from build123d import *

# Parameters (mm, degrees)
SKETCH_1_R          = 30
EXTRUDE_1_DEPTH     = 10
SKETCH_2_R          = 40
EXTRUDE_2_DEPTH     = 60
CUT_EXTRUDE_START   = -40
SKETCH_3_R          = 75
CUT_EXTRUDE_1_DEPTH = 40
CUT_EXTRUDE_2_DEPTH = 10


with BuildPart() as part:
    # Sketch 1 → Extrude 1 (new body)
    with BuildSketch(Plane(origin=(0, 0, 0), x_dir=(1, 0, 0), z_dir=(0, 1, 0))):
        with BuildLine():
            Line((-500, -450), (500, -450))
            ThreePointArc((500, -450), (570.710678119, -420.710678119), (600, -350))
            Line((600, -350), (600, 350))
            ThreePointArc((600, 350), (570.710678119, 420.710678119), (500, 450))
            Line((500, 450), (-500, 450))
            ThreePointArc((-500, 450), (-570.710678119, 420.710678119), (-600, 350))
            Line((-600, 350), (-600, -350))
            ThreePointArc((-600, -350), (-570.710678119, -420.710678119), (-500, -450))
        make_face()
        with Locations(Location((-500, 350, 0), (0, 0, 270))):
            Circle(SKETCH_1_R, mode=Mode.SUBTRACT)
        with Locations(Location((500, 350, 0), (0, 0, 270))):
            Circle(SKETCH_1_R, mode=Mode.SUBTRACT)
        with Locations(Location((-500, -350, 0), (0, 0, 270))):
            Circle(SKETCH_1_R, mode=Mode.SUBTRACT)
        with Locations(Location((500, -350, 0), (0, 0, 270))):
            Circle(SKETCH_1_R, mode=Mode.SUBTRACT)
    extrude(amount=EXTRUDE_1_DEPTH)

    # Sketch 2 → Extrude 2 (add)
    with BuildSketch(Plane(origin=(0, 10, 0), x_dir=(1, 0, 0), z_dir=(0, 1, 0))):
        with BuildLine():
            Line((600, -350), (600, 350))
            ThreePointArc((600, 350), (570.710678119, 420.710678119), (500, 450))
            Line((500, 450), (-500, 450))
            ThreePointArc((-500, 450), (-570.710678119, 420.710678119), (-600, 350))
            Line((-600, 350), (-600, -350))
            ThreePointArc((-600, -350), (-570.710678119, -420.710678119), (-500, -450))
            Line((-500, -450), (500, -450))
            ThreePointArc((500, -450), (570.710678119, -420.710678119), (600, -350))
        make_face()
        with Locations(Location((-500, 350, 0), (0, 0, 270))):
            Circle(SKETCH_2_R, mode=Mode.SUBTRACT)
        with Locations(Location((-500, -350, 0), (0, 0, 270))):
            Circle(SKETCH_2_R, mode=Mode.SUBTRACT)
        with Locations(Location((500, -350, 0), (0, 0, 270))):
            Circle(SKETCH_2_R, mode=Mode.SUBTRACT)
        with Locations(Location((500, 350, 0), (0, 0, 270))):
            Circle(SKETCH_2_R, mode=Mode.SUBTRACT)
    extrude(amount=EXTRUDE_2_DEPTH)

    # Sketch 3 → Cut-Extrude 1 (cut)
    with BuildSketch(Plane(origin=(0, 70, 0), x_dir=(1, 0, 0), z_dir=(0, 1, 0)).offset(CUT_EXTRUDE_START)):
        with BuildLine():
            Line((600, -350), (600, 350))
            ThreePointArc((600, 350), (570.710678119, 420.710678119), (500, 450))
            Line((500, 450), (-500, 450))
            ThreePointArc((-500, 450), (-570.710678119, 420.710678119), (-600, 350))
            Line((-600, 350), (-600, -350))
            ThreePointArc((-600, -350), (-570.710678119, -420.710678119), (-500, -450))
            Line((-500, -450), (500, -450))
            ThreePointArc((500, -450), (570.710678119, -420.710678119), (600, -350))
        make_face()
        with Locations(Location((-500, 350, 0), (0, 0, 270))):
            Circle(SKETCH_3_R, mode=Mode.SUBTRACT)
        with Locations(Location((-500, -350, 0), (0, 0, 270))):
            Circle(SKETCH_3_R, mode=Mode.SUBTRACT)
        with Locations(Location((500, 350, 0), (0, 0, 270))):
            Circle(SKETCH_3_R, mode=Mode.SUBTRACT)
        with Locations(Location((500, -350, 0), (0, 0, 270))):
            Circle(SKETCH_3_R, mode=Mode.SUBTRACT)
    extrude(amount=CUT_EXTRUDE_1_DEPTH, mode=Mode.SUBTRACT)

    # Sketch 7 → Cut-Extrude 2 (cut)
    with BuildSketch(Plane(origin=(0, 70, 0), x_dir=(1, 0, 0), z_dir=(0, 1, 0))):
        with BuildLine():
            Line((-425, 346.5), (-445, 346.5))
            ThreePointArc((-445, 346.5), (-448.5, 350), (-445, 353.5))
            Line((-445, 353.5), (-425, 353.5))
            ThreePointArc((-425, 353.5), (-421.5, 350), (-425, 346.5))
        make_face()
        with BuildLine():
            Line((575, 346.5), (555, 346.5))
            ThreePointArc((555, 346.5), (551.5, 350), (555, 353.5))
            Line((555, 353.5), (575, 353.5))
            ThreePointArc((575, 353.5), (578.5, 350), (575, 346.5))
        make_face()
        with BuildLine():
            Line((575, -353.5), (555, -353.5))
            ThreePointArc((555, -353.5), (551.5, -350), (555, -346.5))
            Line((555, -346.5), (575, -346.5))
            ThreePointArc((575, -346.5), (578.5, -350), (575, -353.5))
        make_face()
        with BuildLine():
            Line((-425, -353.5), (-445, -353.5))
            ThreePointArc((-445, -353.5), (-448.5, -350), (-445, -346.5))
            Line((-445, -346.5), (-425, -346.5))
            ThreePointArc((-425, -346.5), (-421.5, -350), (-425, -353.5))
        make_face()
    extrude(amount=-CUT_EXTRUDE_2_DEPTH, mode=Mode.SUBTRACT)


solid = part.part
Can you work these out from the model? Positions are in its coordinate system, mm. A direction names the side the tool comes from. Coordinates: 2 decimals unless noted, no trailing zeros. Write each loop counter-clockwise with the first axis right and the second up, starting at its lowest first coordinate (ties: lowest second). Pieces come first, ordered by that corner, then holes. Notation, with made-up numbers: (33, 65.5) - (73, 65.5) arc R11 cw to (73, 70.5) - close; hole circle Ø7 at (-33, 1). An arc over 180 degrees is marked (long way). Return JSON: item names as keys, results as strings. Group by question number.
Item 1: If we section it at D-D (z = 29): Write out the boundary of the cut face in (x, y).
Item 2: Which directions (+Z, -Z, +X, -X, +Y, -Y) give clear straight access to the entire face, cutting with the end or side of a thin tool? Please do faces 5 (the face through (-600, 15, -5)), 6 (the face through (563.24, 49.72, -309.68)).
Item 3: We'd pull the mould along X, two halves only. Please class faces 1 (the face through (-571.484, 14.79, 419.929)), 2 (the face through (-529.287, 4.93, 343.497)), 3 (the face through (571.484, 14.79, -419.929)), 4 (the face through (-7, 15, 450)): pulls with the +X half, pulls with the -X half, needs draft (parallel to the pull), parting line crosses it, or undercut.
Item 4: If we section it at B-B (z = 366): Write out the boundary of the cut face in (x, y), then the cut area to 3 significant figures.
Item 5: If we section it at A-A (y = 48): Write out the boundary of the cut face in (x, z).
Item 6: Please list where these lines run through material, in increasing order: probe 1 along X at (y, z) = (5.25, -350); probe 2 along X at (y, z) = (53, 350); probe 3 along X at (y, z) = (23, -350).
Item 7: I'm going to push flat-ended pins straight in: pin 1 Ø11 at (x, y) = (-432.5, 63) entering from -Z; pin 2 Ø8 at (x, z) = (299.5, -59.5) entering from +Y; pin 3 Ø10 at (y, z) = (39, -180) entering from +X; pin 4 Ø3 at (x, y) = (561.5, 63) entering from -Z. Where does each tip first touch, or does it pass through?
Item 8: If we section it at C-C (x = -39): Write out the boundary of the cut face in (y, z), then the cut area to 3 significant figures.
Return value:
{
 "1": {"outline": "(-600, 0) - (600, 0) - (600, 30) - (-600, 30) - close"},
 "2": {"face 5": "+Z, -Z, -X, +Y, -Y", "face 6": "+Y"},
 "3": {"face 1": "pulls with the -X half", "face 2": "undercut", "face 3": "pulls with the +X half", "face 4": "needs draft"},
 "4": {"outline": "(-598.71, 0) - (-525.38, 0) - (-525.38, 10) - (-536.66, 10) - (-536.66, 70) - (-573.27, 70) - (-573.27, 30) - (-598.71, 30) - close; (-474.62, 0) - (474.62, 0) - (474.62, 10) - (463.34, 10) - (463.34, 70) - (426.73, 70) - (426.73, 30) - (-426.73, 30) - (-426.73, 70) - (-463.34, 70) - (-463.34, 10) - (-474.62, 10) - close; (525.38, 0) - (598.71, 0) - (598.71, 30) - (573.27, 30) - (573.27, 70) - (536.66, 70) - (536.66, 10) - (525.38, 10) - close", "area": "37,800 mm^2"},
 "5": {"outline": "circle Ø150 at (-500, -350); circle Ø150 at (-500, 350); circle Ø150 at (500, -350); circle Ø150 at (500, 350); hole circle Ø80 at (-500, -350); hole circle Ø80 at (-500, 350); hole circle Ø80 at (500, -350); hole circle Ø80 at (500, 350)"},
 "6": {"probe 1": "x = -600 to -530, -470 to 470, 530 to 600", "probe 2": "x = -575 to -540, -460 to -425, 425 to 460, 540 to 575", "probe 3": "x = -600 to -540, -460 to 460, 540 to 600"},
 "7": {"pin 1": "stops at z = -392.2", "pin 2": "stops at y = 30", "pin 3": "passes through", "pin 4": "stops at z = -395"},
 "8": {"outline": "(0, -450) - (30, -450) - (30, 450) - (0, 450) - close", "area": "27,000 mm^2"}
}
